```python
from build123d import *

# Parameters (mm, degrees)
BOSS_EXTRUDE1_DEPTH = 32
SKETCH2_R           = 9.5
CUT_EXTRUDE1_DEPTH  = 98.205966895
SKETCH3_R           = 34
CUT_EXTRUDE2_DEPTH  = 20
CUT_EXTRUDE3_START  = -20
CUT_EXTRUDE3_DEPTH  = 20
SKETCH5_R           = 4.5
CUT_EXTRUDE4_DEPTH  = 3
SKETCH6_R           = 3
CUT_EXTRUDE5_DEPTH  = 104.865297412


# Read off the part's stored shape, not the designer's step: Cut-Extrude3
with BuildPart() as part:
    # Sketch1 → Boss-Extrude1 (new, symmetric)
    with BuildSketch(Plane.XY):
        with BuildLine():
            Line((32, 0), (36, 0))
            Line((36, 0), (36, 25))
            Line((36, 25), (80, 25))
            Line((80, 25), (80, 45))
            Line((80, 45), (36.592348927, 45))
            ThreePointArc((36.592348927, 45), (19.416487839, 54.653453688), (0, 58))
            Line((0, 58), (0, 32))
            ThreePointArc((0, 32), (22.627416998, 22.627416998), (32, 0))
        make_face()
    boss_extrude1 = extrude(amount=BOSS_EXTRUDE1_DEPTH, both=True)

    # Sketch2 → Cut-Extrude1 (cut, through all)
    with BuildSketch(Plane(origin=(0, 45, 0), x_dir=(1, 0, 0), z_dir=(0, 1, 0))):
        with Locations(Location((52.5, 0, 0), (0, 0, 180))):
            Circle(SKETCH2_R)
    cut_extrude1 = extrude(amount=-CUT_EXTRUDE1_DEPTH, mode=Mode.SUBTRACT)

    # Sketch3 → Cut-Extrude2 (cut, symmetric)
    with BuildSketch(Plane.XY):
        Circle(SKETCH3_R)
    cut_extrude2 = extrude(amount=CUT_EXTRUDE2_DEPTH, both=True, mode=Mode.SUBTRACT)

    # Cut-Extrude3 outline → Cut-Extrude3 (cut)
    with BuildSketch(Plane(origin=(0, 45, 0), x_dir=(1, 0, 0), z_dir=(0, 1, 0)).offset(CUT_EXTRUDE3_START)):
        with BuildLine():
            ThreePointArc((73.321211119, 32), (78.312505014, 16.344771592), (80, 1.98e-07))
            Line((80, 1.98e-07), (80, 32))
            Line((80, 32), (73.321211119, 32))
        make_face()
        with BuildLine():
            ThreePointArc((80, 1.98e-07), (78.312505055, -16.344771398), (73.321211119, -32))
            Line((73.321211119, -32), (80, -32))
            Line((80, -32), (80, 1.98e-07))
        make_face()
    cut_extrude3 = extrude(amount=CUT_EXTRUDE3_DEPTH, mode=Mode.SUBTRACT)

    # Mirror1: Boss-Extrude1, Cut-Extrude1, Cut-Extrude2, Cut-Extrude3 across plane
    add(boss_extrude1.mirror(Plane(origin=(0, 32, 32), x_dir=(0, 0, 1), z_dir=(1, 0, 0))))
    add(cut_extrude1.mirror(Plane(origin=(0, 32, 32), x_dir=(0, 0, 1), z_dir=(1, 0, 0))), mode=Mode.SUBTRACT)
    add(cut_extrude2.mirror(Plane(origin=(0, 32, 32), x_dir=(0, 0, 1), z_dir=(1, 0, 0))), mode=Mode.SUBTRACT)
    add(cut_extrude3.mirror(Plane(origin=(0, 32, 32), x_dir=(0, 0, 1), z_dir=(1, 0, 0))), mode=Mode.SUBTRACT)

    # Sketch5 → Cut-Extrude4 (cut)
    with BuildSketch(Plane(origin=(0, 58, 0), x_dir=(1, 0, 0), z_dir=(0, 1, 0))):
        with Locations(Location((0, 0, 0), (0, 0, 270))):
            Circle(SKETCH5_R)
    extrude(amount=-CUT_EXTRUDE4_DEPTH, mode=Mode.SUBTRACT)

    # Sketch6 → Cut-Extrude5 (cut, through all)
    with BuildSketch(Plane(origin=(0, 58, 0), x_dir=(1, 0, 0), z_dir=(0, 1, 0))):
        with Locations(Location((0, 0, 0), (0, 0, 270))):
            Circle(SKETCH6_R)
    extrude(amount=-CUT_EXTRUDE5_DEPTH, mode=Mode.SUBTRACT)


solid = part.part
```
Work out the finished part from the listing and answer in its coordinate system (mm). A direction names the side the tool comes from. Give positions to 0.01 mm unless a question says otherwise; leave off trailing zeros. Order: outer loops, then holes, each group sorted by start corner. A loop starts at its lowest first (then second) coordinate and runs counter-clockwise, first axis right, second up. Notation, with made-up numbers: (0.5, 52.5) - (48.5, 52.5) arc R23 ccw to (48.5, 76.5) - close; hole circle Ø3 at (-20, -19.5). An arc over 180 degrees is marked (long way). One line per item, written item: value. Start each with the question number.
1. Section C-C, the plane y = 38 is taken. Write down the section's boundary in (x, z), then the cut area to 3 significant figures.
2. Section D-D, the plane z = 27.5 is taken. Write down the section's boundary in (x, y), then the cut area to 3 significant figures.
3. Which of the six approach directions +Z, -Z, +X, -X, +Y, -Y give full straight-line access (tool end or side, diameter ignored) to faces 4 (the face through (0.2, 32.2, -20)), 5 (the face through (-63, 45, 0)), 6 (the face through (-63, 25, 0))?
4. Section B-B, the plane y = 12.5 is taken. Write down the section's boundary in (x, z), then the cut area to 3 significant figures.
5. Consider line 1 (Z direction, x = 0, y = 40); line 2 (X direction, y = 38, z = -7.5); line 3 (Z direction, x = 52, y = 31). Determine where each line is inside the solid, lowest interval first.
6. Section A-A, the plane x = 52.5 is taken. Write down the section's boundary in (y, z).
7. Each of these flat-tipped pins is pushed along its axis until it touches: pin 1 Ø1 at (y, z) = (25.5, -23.5) entering from +X; pin 2 Ø6 at (y, z) = (49, -11.5) entering from -X; pin 3 Ø1 at (y, z) = (22.5, 2) entering from -X; pin 4 Ø17 at (x, z) = (52.5, 0) entering from +Y. Where does it stop, or does it pass through?
8. For a pull along Z with two mould halves and no side action, classify faces 1 (the face through (-3, 55, 1)), 2 (the face through (1, 36, 32)), 3 (the face through (63, 45, 0)) as released by +Z, released by -Z, zero draft, split by the parting line, or undercut.
Filled sheet:
1. outline: (-73.32, -32) - (73.32, -32) arc R80 ccw to (73.32, 32) - (-73.32, 32) arc R80 ccw to start; hole circle Ø19 at (-52.5, 0); hole circle Ø6 at (0, 0); hole circle Ø19 at (52.5, 0)
1. area: 9,360 mm²
2. outline: (-75.12, 25) - (-36, 25) - (-36, 0) - (-32, 0) arc R32 cw to (32, 0) - (36, 0) - (36, 25) - (75.12, 25) - (75.12, 45) - (36.59, 45) arc R58 ccw to (-36.59, 45) - (-75.12, 45) - close
2. area: 3,850 mm²
3. face 4: -Y
3. face 5: +Z, -Z, -X, +Y
3. face 6: +Z, -Z, -X, -Y
4. outline: (-36, -32) - (-29.46, -32) - (-29.46, -20) - (-31.62, -20) - (-31.62, 20) - (-29.46, 20) - (-29.46, 32) - (-36, 32) - close; (29.46, -32) - (36, -32) - (36, 32) - (29.46, 32) - (29.46, 20) - (31.62, 20) - (31.62, -20) - (29.46, -20) - close
4. area: 665 mm²
5. line 1: -32 to -3, 3 to 32
5. line 2: -79.65 to -58.33, -46.67 to 46.67, 58.33 to 79.65
5. line 3: -32 to -9.49, 9.49 to 32
6. outline: (25, -32) - (45, -32) - (45, -9.5) - (25, -9.5) - close; (25, 9.5) - (45, 9.5) - (45, 32) - (25, 32) - close
7. pin 1: x = 76.62
7. pin 2: x = -35.33
7. pin 3: x = -36
7. pin 4: through
8. face 1: undercut
8. face 2: released by +Z
8. face 3: zero draft
